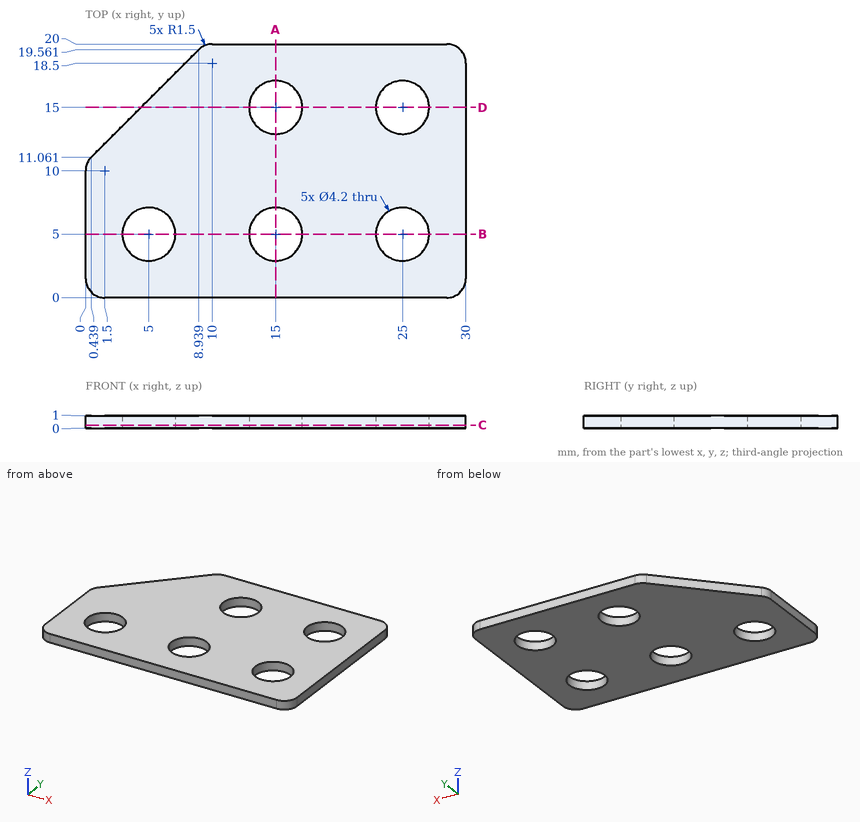
Could you check a few things on this drawing? It's one solid part, dimensions in mm from its lowest x, y, z. Round coordinates to 2 decimals unless told otherwise and drop trailing zeros. Order: outer loops, then holes, each group sorted by start corner. A loop starts at its lowest first (then second) coordinate and runs counter-clockwise, first axis right, second up. Notation, with made-up numbers: (-10, 55) -> (28, 55) arc R18 ccw to (28, 84) -> close; hole circle Ø5 at (16.5, 9). An arc over 180 degrees is marked (long way). One line per question, with ' | ' between items.
Q1. I'm going to push a flat-ended pin straight in: pin 1 (3.5 mm diameter, centred on x = 25, y = 15, fed in from -Z). Where does the tip first touch, or does it pass through?
Computed values:
pin 1: through
Q2. If we section it at B-B on y = 5: Write out the boundary of the cut face in (x, z).
Computed values:
outline: (0, 0) -> (2.9, 0) -> (2.9, 1) -> (0, 1) -> close; (7.1, 0) -> (12.9, 0) -> (12.9, 1) -> (7.1, 1) -> close; (17.1, 0) -> (22.9, 0) -> (22.9, 1) -> (17.1, 1) -> close; (27.1, 0) -> (30, 0) -> (30, 1) -> (27.1, 1) -> close
Q3. If I drill on line 1 (Y direction, x = 25, z = 0.65); line 2 (Y direction, x = 24, z = 0.2); line 3 (X direction, y = 15.75, z = 0.7), over which ranges is the centre line in solid material (lowest first)? Write a range as from..to.
Computed values:
line 1: 0..2.9, 7.1..12.9, 17.1..20 | line 2: 0..3.15, 6.85..13.15, 16.85..20 | line 3: 5.13..13.04, 16.96..23.04, 26.96..30
Q4. If we section it at C-C on z = 0.25: Write out the boundary of the cut face in (x, y), plus the area to 3 significant figures.
Computed values:
outline: (0, 1.5) arc R1.5 ccw to (1.5, 0) -> (28.5, 0) arc R1.5 ccw to (30, 1.5) -> (30, 18.5) arc R1.5 ccw to (28.5, 20) -> (10, 20) arc R1.5 ccw to (8.94, 19.56) -> (0.44, 11.06) arc R1.5 ccw to (0, 10) -> close; hole circle Ø4.2 at (5, 5); hole circle Ø4.2 at (15, 5); hole circle Ø4.2 at (15, 15); hole circle Ø4.2 at (25, 5); hole circle Ø4.2 at (25, 15) | area: 485 mm²
Q5. If we section it at A-A on x = 15: Write out the boundary of the cut face in (y, z), plus the area to 3 significant figures.
Computed values:
outline: (0, 0) -> (2.9, 0) -> (2.9, 1) -> (0, 1) -> close; (7.1, 0) -> (12.9, 0) -> (12.9, 1) -> (7.1, 1) -> close; (17.1, 0) -> (20, 0) -> (20, 1) -> (17.1, 1) -> close | area: 11.6 mm²
Q6. If we section it at D-D on y = 15: Write out the boundary of the cut face in (x, z), plus the area to 3 significant figures.
Computed values:
outline: (4.38, 0) -> (12.9, 0) -> (12.9, 1) -> (4.38, 1) -> close; (17.1, 0) -> (22.9, 0) -> (22.9, 1) -> (17.1, 1) -> close; (27.1, 0) -> (30, 0) -> (30, 1) -> (27.1, 1) -> close | area: 17.2 mm²
